Check sheet for the modelled part. Datum: model origin and axes. Units: mm. A direction names the side the tool comes from. Give positions to 0.01 mm unless a question says otherwise; leave off trailing zeros. Loops run counter-clockwise (first coordinate to the right, second up) from the corner with the lowest first, then second, coordinate; pieces in that order, holes last. Notation, with made-up numbers: M 23.5,-13 L 31.5,-13 A12 cw 31.5,-4 Z; hole C 32,77.25 d9. An arc over 180 degrees is marked long. Use one line per item in the form item = value.
Autodesk Inventor part; units mm, degrees
ref_plane "YZ Plane" through (0, 0, 0) normal (1, 0, 0) x (0, 1, 0)
ref_plane "XZ Plane" through (0, 0, 0) normal (0, 1, 0) x (-1, 0, 0)
ref_plane "XY Plane" through (0, 0, 0) normal (0, 0, 1) x (1, 0, 0)
sketch "Sketch1" plane through (0, 0, 0) normal (0, 0, 1) x (1, 0, 0)
  circle A0 centre (-2.5, -3) radius 1.6
  line L0 (-10, -5.75) -> (0, -5.75)
  line L1 (0, 0) -> (0, -5.75)
  line L2 (-10, 0) -> (0, 0)
  line L3 (-10, -1.75) -> (-10, 0)
  line L4 (-10, -5.75) -> (-10, -4.05)
  line L5 (0, -5.75) -> (-5, -5.75)
  line L6 (-5, -5.75) -> (-5, 0)
  line L7 (-5, 0) -> (0, 0)
  line L8 (0, 0) -> (0, -5.75)
  line L9 (-10, -1.75) -> (-9.2455, -1.75)
  line L10 (-9.2455, -1.75) -> (-9.2455, -4.05)
  line L11 (-9.2455, -4.05) -> (-10, -4.05)
  dimension "d0" = 2.5
extrude "Extrusion1" add sketch "Sketch1" along normal blind 4 contours L6 L2 L1 L0
sketch "Sketch2" plane through (-5, 0, 0) normal (0, 1, 0) x (1, 0, 0)
  line L0 (5, 0) -> (0, 0)
  line L1 (0, 0) -> (0, -4)
  line L2 (5, -4) -> (0, -4)
  line L3 (5, 0) -> (5, -4)
  line L4 (24.0211, -5.907) -> (18.6171, -5.907)
  line L5 (24.0211, -17.407) -> (18.6171, -17.407)
  line L6 (5, -4) -> (18.0171, -13.657)
  line L7 (5, 0) -> (18.0171, -9.657)
  line L8 (18.6171, -17.407) -> (18.6171, -13.657) construction
  line L9 (18.6171, -5.907) -> (18.6171, -9.657) construction
  line L10 (18.6171, -9.657) -> (18.6171, -13.657) construction
  line L11 (24.0211, -5.907) -> (24.0211, -17.407) construction
  line L12 (18.0171, -9.657) -> (26.5171, -9.657)
  line L13 (18.0171, -13.657) -> (26.5171, -13.657)
  line L14 (26.5171, -13.657) -> (26.5171, -9.657)
  line L15 (20.0171, -11.057) -> (20.0171, -5.657) construction
  point P0 (24.0211, -11.657)
  point P1 (18.6171, -11.657)
  dimension "d3" = 4
  dimension "d4" = 8.5
  dimension "d7" = 2
extrude "Extrusion2" add sketch "Sketch2" against normal blind 10 contours L7 L12 L14 L13 L6 L3
sketch "Sketch3" plane through (13.0171, 0, 13.657) normal (0, 0, 1) x (1, 0, 0)
  circle A0 centre (4.6, -6.8) radius 1.55 construction
  line L0 (-13.0171, 0) -> (0, 0) construction
  line L1 (-13.0171, -5.75) -> (-13.0171, 0)
  line L2 (-13.0171, -5.75) -> (-13.0171, -10)
  line L3 (0, -10) -> (-13.0171, -10)
  line L4 (0, 0) -> (0, -10) construction
  line L5 (0, 0) -> (8.5, 0)
  line L6 (0, 0) -> (0, -10) construction
  line L7 (8.5, -10) -> (0, -10) construction
  line L8 (8.5, 0) -> (8.5, -10)
  line L9 (-18.0171, -5.75) -> (-13.0171, -5.75)
  line L10 (-13.0171, -5.75) -> (-9.0171, -5.75)
  line L11 (-9.0171, -5.75) -> (1.6, -10)
  line L12 (8.5, -10) -> (0, -10)
  line L13 (-13.0171, 0) -> (-18.0171, 0)
  line L14 (-13.0171, 0) -> (-9.0171, 0)
  line L15 (0, 0) -> (-13.0171, 0)
  line L16 (-9.0171, 0) -> (1.6, -4.25)
  line L17 (1.6, -4.25) -> (7.6, -4.25)
  line L18 (7.6, -4.25) -> (7.6, -10)
  line L19 (2.7105, -10) -> (7.6, -10)
  dimension "d8" = 4
  dimension "d9" = 4
  dimension "d11" = 3
  dimension "d12" = 3
extrude "Extrusion3" cut sketch "Sketch3" against normal through all contours L10 L11 L12 L3 L2 | L15 L5 L8 L12 L18 L17 L16
sketch "Sketch4" plane through (14.6171, -10, 13.657) normal (0, 0, 1) x (1, 0, 0)
  line L0 (-1.6, 0.6405) -> (0, 0)
  line L1 (6, 0) -> (0, 0)
  line L2 (6, 0) -> (6, 5.75)
  line L3 (6, 5.75) -> (0, 5.75)
  line L4 (0, 5.75) -> (-1.6, 6.3905)
  line L5 (-1.6, 6.3905) -> (-1.6, 0.6405)
  circle A0 centre (3, 3.2) radius 1.55
  point P0 (-14.6171, 10)
extrude "Extrusion4" cut sketch "Sketch4" against normal through all contours A0
properties part number "Palanca servo_dedo_2"
1) Section check B-B (y = -6). Record the cut outline in (x, z), then the cut area to 3 significant figures.
Evaluation:
outline = M 4.62,3.43 L 13.02,9.66 L 16.29,9.66 L 16.29,13.66 L 13.02,13.66 L 4.62,7.43 Z; M 18.94,9.66 L 20.62,9.66 L 20.62,13.66 L 18.94,13.66 Z
area = 53.3 mm^2
2) Scan lines: line 1 (Y direction, x = -2.5, z = 0.95); line 2 (X direction, y = -6, z = 10.5); line 3 (Z direction, x = -0.25, y = -1). Record each from-to range of solid material in increasing order.
Evaluation:
line_1 = -5.75 to -4.6, -1.4 to 0
line_2 = 8.76 to 16.29, 18.94 to 20.62
line_3 = 0 to 4
3) Depth check by flat-ended pin: pin 1 Ø2 at (x, y) = (5, -3.5) entering from +Z; pin 2 Ø2 at (x, y) = (10, -3) entering from -Z; pin 3 Ø2 at (x, z) = (1, 4.5) entering from -Y. Enter the tip coordinate at first touch or a pass-through.
Evaluation:
pin_1 = 8.45
pin_2 = 6.68
pin_3 = -5.75
4) Release check for a two-part mould opening along Y. For faces 4 (the face through (17.415, -5.263, 11.685)), 5 (the face through (20.617, -7, 12)), 6 (the face through (9.234, -7.845, 8.387)), 7 (the face through (-2.85, -1.44, 1.97)) record: pulls with the +Y half, pulls with the -Y half, needs draft (parallel to the pull), parting line crosses it, or undercut.
Evaluation:
face_4 = undercut
face_5 = needs draft
face_6 = pulls with the -Y half
face_7 = undercut
5) Section check C-C (y = -2.25). Record the cut outline in (x, z).
Evaluation:
outline = M -5,0 L -3.91,0 L -3.91,4 L -5,4 Z; M -1.09,0 L 0,0 L 9.62,7.14 L 9.62,11.14 L 0,4 L -1.09,4 Z
6) Section check D-D (x = 5.75). Record the cut outline in (y, z).
Evaluation:
outline = M -6.45,4.27 L -0.7,4.27 L -0.7,8.27 L -6.45,8.27 Z
7) Set-up check for faces 1 (the face through (-1, -2, 4)), 2 (the face through (18, -4.25, 12)), 3 (the face through (-1, -5.75, 3)): record each of +Z, -Z, +X, -X, +Y, -Y from which the full face is reachable in a straight line by a thin tool's end or side.
Evaluation:
face_1 = +Z, -X, +Y, -Y
face_2 = +Z, -Z, +X, +Y
face_3 = +Z, -Z, -X, -Y
8) Section check A-A (x = -2.5). Record the cut outline in (y, z).
Evaluation:
outline = M -5.75,0 L -4.6,0 L -4.6,4 L -5.75,4 Z; M -1.4,0 L 0,0 L 0,4 L -1.4,4 Z
